```python
from build123d import *

# Parameters (mm, degrees)
SKETCH1_W               = 20
SKETCH1_H               = 12.5
BOSS_EXTRUDE2_DEPTH     = 5
CUT_EXTRUDE6_DEPTH      = 131.001332273
CUT_EXTRUDE2_DEPTH      = 130.239475323
CUT_EXTRUDE2_DEPTH_BACK = 130.239475323
SKETCH2_R               = 1.75
SKETCH2_3_R             = 3.5
SKETCH2_3_R_2           = 1.75
CUT_EXTRUDE4_DEPTH      = 3.5


with BuildPart() as part:
    # Sketch1 → Boss-Extrude2 (new body)
    with BuildSketch(Plane.XY):
        Polygon((10, 77.5), (10, 22.5), (77.847550572, 22.5), (93.676818865, 50), (77.847550572, 77.5), align=None)
        with Locations((45.4, 83.75)):
            Rectangle(SKETCH1_W, SKETCH1_H)
        with Locations((45.4, 16.25)):
            Rectangle(SKETCH1_W, SKETCH1_H)
    extrude(amount=BOSS_EXTRUDE2_DEPTH)

    # Sketch6 → Cut-Extrude6 (cut, through all)
    with BuildSketch(Plane.XY):
        Polygon((35.4, 10), (55.4, 10), (55.4, 22.5), (77.847550572, 22.5), (93.676818865, 50), (77.847550572, 77.5), (55.4, 77.5), (55.4, 90), (35.4, 90), (35.4, 77.5), (10, 77.5), (10, 22.5), (35.4, 22.5), align=None)
        Polygon((54.9, 10.5), (54.9, 23), (77.558439817, 23), (93.099903232, 50), (77.558439817, 77), (54.9, 77), (54.9, 89.5), (35.9, 89.5), (35.9, 77), (10.5, 77), (10.5, 23), (35.9, 23), (35.9, 10.5), align=None, mode=Mode.SUBTRACT)
    extrude(amount=CUT_EXTRUDE6_DEPTH, mode=Mode.SUBTRACT)

    # Sketch2 → Cut-Extrude2 (cut, two sides: drawn at the far end of the back side and taken through both)
    with BuildSketch(Plane.XY.offset(-CUT_EXTRUDE2_DEPTH_BACK)):
        with Locations((45.4, 83.75)):
            Circle(SKETCH2_R)
        with Locations((45.4, 16.25)):
            Circle(SKETCH2_R)
    extrude(amount=CUT_EXTRUDE2_DEPTH + CUT_EXTRUDE2_DEPTH_BACK, mode=Mode.SUBTRACT)

    # Sketch2_3 → Cut-Extrude4 (cut)
    # profile 1 of 2: a face of its own
    with BuildSketch(Plane.XY):
        with Locations(Location((45.4, 83.75, 0), (0, 0, 180))):
            Circle(SKETCH2_3_R)
        with Locations((45.4, 83.75)):
            Circle(SKETCH2_3_R_2, mode=Mode.SUBTRACT)
    # profile 2 of 2: a face of its own
    with BuildSketch(Plane.XY):
        with Locations(Location((45.4, 16.25, 0), (0, 0, 180))):
            Circle(SKETCH2_3_R)
        with Locations((45.4, 16.25)):
            Circle(SKETCH2_3_R_2, mode=Mode.SUBTRACT)
    extrude(amount=CUT_EXTRUDE4_DEPTH, mode=Mode.SUBTRACT)


solid = part.part
```
Verification items for the finished model (mm, model axes). A direction names the side the tool comes from. Coordinates: 2 decimals unless noted, no trailing zeros. Loops run counter-clockwise (first coordinate to the right, second up) from the corner with the lowest first, then second, coordinate; pieces in that order, holes last. Notation, with made-up numbers: (-4, -26) - (31, -26) arc R24 cw to (31, 2) - close; hole circle Ø5 at (59.25, 38). An arc over 180 degrees is marked (long way). Put each result on its own line as item: value.
Item 1: Scan lines: line 1 along Y through (x, z) = (45.4, 1.45); line 2 along Y through (x, z) = (45.4, 4.45); line 3 along X through (y, z) = (16.25, 1.7). Record each from-to range of solid material in increasing order.
Conclusion:
line 1: y = 10.5 to 12.75, 19.75 to 80.25, 87.25 to 89.5
line 2: y = 10.5 to 14.5, 18 to 82, 85.5 to 89.5
line 3: x = 35.9 to 41.9, 48.9 to 54.9
Item 2: Gauge pin test, flat ends, axial feed: pin 1 Ø4 at (x, y) = (45.4, 16.25) entering from -Z; pin 2 Ø2.5 at (x, z) = (71, 1.5) entering from +Y; pin 3 Ø3 at (x, z) = (60.5, 1.5) entering from -Y. Record the tip position at first contact, or that the pin passes through.
Conclusion:
pin 1: stops at z = 3.5
pin 2: stops at y = 77
pin 3: stops at y = 23
Item 3: Set-up check for faces 1 (the face through (43.9, 85.3, 3.5)), 2 (the face through (23, 23, 2)), 3 (the face through (23, 77, 2)): record each of +Z, -Z, +X, -X, +Y, -Y from which the full face is reachable in a straight line by a thin tool's end or side.
Conclusion:
face 1: -Z
face 2: +Z, -Z, -X, -Y
face 3: +Z, -Z, -X, +Y
Item 4: Section check C-C (y = 16.25). Enter the section's corners in (x, z), then the cut area to 4 significant figures.
Conclusion:
outline: (35.9, 0) - (41.9, 0) - (41.9, 3.5) - (43.65, 3.5) - (43.65, 5) - (35.9, 5) - close; (47.15, 3.5) - (48.9, 3.5) - (48.9, 0) - (54.9, 0) - (54.9, 5) - (47.15, 5) - close
area: 65.25 mm2
Item 5: Section check B-B (x = 45.4). Enter the section's corners in (y, z).
Conclusion:
outline: (10.5, 0) - (12.75, 0) - (12.75, 3.5) - (14.5, 3.5) - (14.5, 5) - (10.5, 5) - close; (18, 3.5) - (19.75, 3.5) - (19.75, 0) - (80.25, 0) - (80.25, 3.5) - (82, 3.5) - (82, 5) - (18, 5) - close; (85.5, 3.5) - (87.25, 3.5) - (87.25, 0) - (89.5, 0) - (89.5, 5) - (85.5, 5) - close
Item 6: Section check D-D (x = 23.5). Enter the section's corners in (y, z).
Conclusion:
outline: (23, 0) - (77, 0) - (77, 5) - (23, 5) - close
Item 7: Section check A-A (z = 0.85). Enter the section's corners in (x, y), then the cut area to 3 significant figures.
Conclusion:
outline: (10.5, 23) - (35.9, 23) - (35.9, 10.5) - (54.9, 10.5) - (54.9, 23) - (77.56, 23) - (93.1, 50) - (77.56, 77) - (54.9, 77) - (54.9, 89.5) - (35.9, 89.5) - (35.9, 77) - (10.5, 77) - close; hole circle Ø7 at (45.4, 16.25); hole circle Ø7 at (45.4, 83.75)
area: 4,440 mm2
Item 8: Draft check along Y on faces 4 (the face through (85.44, 63.31, 2.46)), 5 (the face through (85.22, 36.31, 2.46)), 6 (the face through (42.167, 17.591, 1.726)). Enter one of: pulls with the +Y half, pulls with the -Y half, needs draft (parallel to the pull), parting line crosses it, or undercut.
Conclusion:
face 4: pulls with the +Y half
face 5: pulls with the -Y half
face 6: undercut
